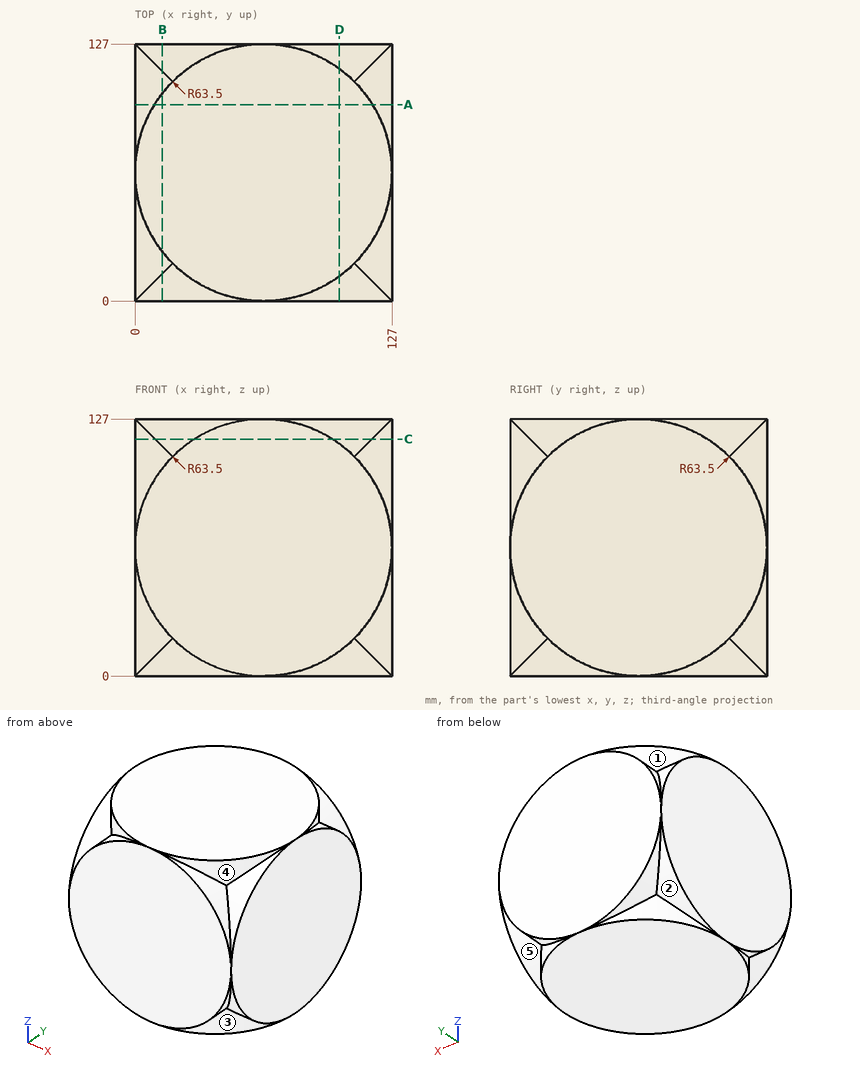
Study the drawing (mm; zero at the part's minimum x, y, z) and answer. A direction names the side the tool comes from. Coordinates: 2 decimals unless noted, no trailing zeros. Order: outer loops, then holes, each group sorted by start corner. A loop starts at its lowest first (then second) coordinate and runs counter-clockwise, first axis right, second up. Notation, with made-up numbers: (63, 23.5) -> (76, 23.5) arc R22 ccw to (76, 41.5) -> close; hole circle Ø5 at (66, 41). An arc over 180 degrees is marked (long way). Answer in a Markdown table with one row per item. Add a question column.
Item 1: Find section B-B (x = 13.5). Write down the section's boundary in (y, z).
Item 2: Find the intervals of material crossed by L1, parallel to X at y = 18, z = 16.5; L2, parallel to Z at x = 121, y = 15; L3, parallel to X at y = 16, z = 107.5, in increasing order. Write a range as from..to.
Item 3: This flat-tipped pin is pushed along its axis until it touches: P1, Ø6, axis at y = 110, z = 50.5, coming from the -X side. Where does it stop, or does it pass through?
Item 4: Find section D-D (x = 101). Write down the section's boundary in (y, z).
Item 5: Find section A-A (y = 97). Write down the section's boundary in (x, z), then the cut area to 3 significant figures.
Item 6: Which of the six approach directions +Z, -Z, +X, -X, +Y, -Y give full straight-line access (tool end or side, diameter ignored) to the marked faces 1, 2, 3, 4 and 5?
Item 7: Find section C-C (z = 117). Write down the section's boundary in (x, y), then the cut area to 3 significant figures.
Result set:
| question | item | result |
|---|---|---|
| 1 | outline | (0, 24.36) -> (13.5, 24.36) arc R63.5 ccw to (24.36, 13.5) -> (24.36, 0) -> (102.64, 0) -> (102.64, 13.5) arc R63.5 ccw to (113.5, 24.36) -> (127, 24.36) -> (127, 102.64) -> (113.5, 102.64) arc R63.5 ccw to (102.64, 113.5) -> (102.64, 127) -> (24.36, 127) -> (24.36, 113.5) arc R63.5 ccw to (13.5, 102.64) -> (0, 102.64) -> close |
| 2 | L1 | x = 19.21..107.79 |
| 2 | L2 | z = 22.51..104.49 |
| 2 | L3 | x = 17.72..109.28 |
| 3 | P1 | stops at x = 0 |
| 4 | outline | (0, 12.26) -> (12.26, 12.26) -> (12.26, 0) -> (114.74, 0) -> (114.74, 12.26) -> (127, 12.26) -> (127, 114.74) -> (114.74, 114.74) -> (114.74, 127) -> (12.26, 127) -> (12.26, 114.74) -> (0, 114.74) -> close |
| 5 | outline | (0, 9.56) -> (9.56, 9.56) -> (9.56, 0) -> (117.44, 0) -> (117.44, 9.56) -> (127, 9.56) -> (127, 117.44) -> (117.44, 117.44) -> (117.44, 127) -> (9.56, 127) -> (9.56, 117.44) -> (0, 117.44) -> close |
| 5 | area | 15,800 mm² |
| 6 | face 1 | +Z, -X, +Y |
| 6 | face 2 | -Z, -X, +Y |
| 6 | face 3 | -Z, +X, -Y |
| 6 | face 4 | +Z, +X, -Y |
| 6 | face 5 | -Z, +X, +Y |
| 7 | outline | (0, 29.29) -> (10, 29.29) arc R63.5 ccw to (29.29, 10) -> (29.29, 0) -> (97.71, 0) -> (97.71, 10) arc R63.5 ccw to (117, 29.29) -> (127, 29.29) -> (127, 97.71) -> (117, 97.71) arc R63.5 ccw to (97.71, 117) -> (97.71, 127) -> (29.29, 127) -> (29.29, 117) arc R63.5 ccw to (10, 97.71) -> (0, 97.71) -> close |
| 7 | area | 13,500 mm² |
